Geometry: final body of the model. Coordinates: model frame, mm. A direction names the side the tool comes from. Coordinates: 2 decimals unless noted, no trailing zeros. Loops run counter-clockwise (first coordinate to the right, second up) from the corner with the lowest first, then second, coordinate; pieces in that order, holes last. Notation, with made-up numbers: (-19.5, 11.5) - (-1.5, 11.5) arc R14 cw to (-1.5, 31.5) - close; hole circle Ø8 at (46.25, 82). An arc over 180 degrees is marked (long way). Return JSON: item names as keys, results as strings.
from build123d import *

# Parameters (mm, degrees)
F1_DEPTH = 1.5
F2_R     = 1
F4_DEPTH = 64
F5_W     = 4.266666
F5_H     = 13.671578
F5_W_2   = 3.2
F6_DEPTH = 7.7216


with BuildPart() as f1:
    # F0 (on Top) → F1 (new body)
    with BuildSketch(Plane.XY):
        with BuildLine():
            Line((32, 7.5), (-32, 7.5))
            Line((-32, 7.5), (-32, -7.5))
            ThreePointArc((-32, -7.5), (0, -4.5), (32, -7.5))
            Line((32, -7.5), (32, 7.5))
        make_face()
    extrude(amount=F1_DEPTH)

    # F2
    f2_edges = [f1.edges().sort_by_distance(p)[0] for p in [
        (32, 7.5, 0.75),
        (32, -7.5, 0.75),
        (-32, -7.5, 0.75),
        (-32, 7.5, 0.75),
    ]]
    fillet(f2_edges, radius=F2_R)

    # F3 (on face) → F4 (join)
    with BuildSketch(Plane.YZ.offset(32)):
        with BuildLine():
            ThreePointArc((1, 1.5), (-1.447266, 3.489226), (0, 6.291288))
            Line((0, 6.291288), (0, 6.803734))
            ThreePointArc((0, 6.803734), (-3.108438, 4.922642), (-4.327623, 1.5))
            Line((-4.327623, 1.5), (1, 1.5))
        make_face()
        with BuildLine():
            ThreePointArc((2, 6.291288), (3.447266, 3.489226), (1, 1.5))
            Line((1, 1.5), (6.5, 1.5))
            ThreePointArc((6.5, 1.5), (5.224821, 4.990141), (2, 6.836136))
            Line((2, 6.836136), (2, 6.291288))
        make_face()
    extrude(amount=-F4_DEPTH)

    # F5 (on face) → F6 (cut)
    with BuildSketch(Plane.XY.offset(1.5)):
        with Locations((0, 2.508166)):
            Rectangle(F5_W, F5_H)
        with Locations((-8, 2.508166)):
            Rectangle(F5_W_2, F5_H)
        with Locations((-14.4, 2.508166)):
            Rectangle(F5_W_2, F5_H)
        with Locations((-20.8, 2.508166)):
            Rectangle(F5_W_2, F5_H)
        with Locations((-27.2, 2.508166)):
            Rectangle(F5_W_2, F5_H)
        with Locations((8, 2.508166)):
            Rectangle(F5_W_2, F5_H)
        with Locations((14.4, 2.508166)):
            Rectangle(F5_W_2, F5_H)
        with Locations((20.8, 2.508166)):
            Rectangle(F5_W_2, F5_H)
        with Locations((27.2, 2.508166)):
            Rectangle(F5_W_2, F5_H)
    extrude(amount=F6_DEPTH, mode=Mode.SUBTRACT)


solid = f1.part
Item 1: Section query C-C, the plane z = 2.25. Count the separate pieces of the cut face and the enclosed holes in it, and give its area (3 significant figures).
Worked out:
{"separate pieces": "20", "enclosed holes": "0", "area": "244 mm^2"}
Item 2: Section query A-A, the plane y = -5.75. Return loops of the section in (x, z), and give its area (3 significant figures).
Worked out:
{"outline": "(-32, 0) - (-20.71, 0) - (-20.71, 1.5) - (-32, 1.5) - close; (20.71, 0) - (32, 0) - (32, 1.5) - (20.71, 1.5) - close", "area": "33.9 mm^2"}
Item 3: Ray query, probe 1 along Z at (x, y) = (11, -4.5); probe 2 along Y at (x, z) = (18, 3); probe 3 along Y at (x, z) = (23, 2). Return the intervals inside material, ascending. Write a range as from..to.
Worked out:
{"probe 1": "0..1.5", "probe 2": "-4.12..-1.29, 3.29..6.29", "probe 3": "-4.3..-0.5, 2.5..6.48"}
Item 4: First-contact query: pin 1 Ø1 at (x, z) = (8.5, 3.5) entering from +Y; pin 2 Ø4 at (x, z) = (2.5, 6) entering from +Y; pin 3 Ø6 at (x, y) = (-13, -2) entering from +Z. Flat tips, straight axial feed; report the tip coordinate or a pass-through.
Worked out:
{"pin 1": "through", "pin 2": "y = 5.89", "pin 3": "z = 6.8"}
Item 5: Section query B-B, the plane x = 3. Return loops of the section in (y, z), and give its area (3 significant figures).
Worked out:
{"outline": "(-4.53, 0) - (7.5, 0) - (7.5, 1.5) - (6.5, 1.5) arc R5.41 ccw to (2, 6.84) - (2, 6.29) arc R2.5 cw (long way) to (0, 6.29) - (0, 6.8) arc R5.41 ccw to (-4.33, 1.5) - (-4.53, 1.5) - close", "area": "43.5 mm^2"}
Item 6: Mould query, pull axis X, two halves, no side actions, for faces 1 (the face through (32, 1, 1)), 2 (the face through (-9.6, 4, 4)), 3 (the face through (24.02, -3.08, 4.96)). Classes: +X half, -X half, draft (parallel to the pull), parting line (faces both ways), or undercut.
Worked out:
{"face 1": "+X half", "face 2": "undercut", "face 3": "draft"}
Item 7: Reachability of faces 4 (the face through (17.62, -3.08, 4.96)), 5 (the face through (28.8, 4, 4)) from +Z, -Z, +X, -X, +Y, -Y: full face, straight path, thin tool, end or side. Return the list, or none.
Worked out:
{"face 4": "+Z, +X, -X, -Y", "face 5": "+Z, +Y, -Y"}
Item 8: Section query D-D, the plane x = -4.5. Return loops of the section in (y, z).
Worked out:
{"outline": "(-4.56, 0) - (7.5, 0) - (7.5, 1.5) - (6.5, 1.5) arc R5.41 ccw to (2, 6.84) - (2, 6.29) arc R2.5 cw (long way) to (0, 6.29) - (0, 6.8) arc R5.41 ccw to (-4.33, 1.5) - (-4.56, 1.5) - close"}
